from build123d import *

# Parameters (mm, degrees)
SKETCH1_R           = 1.778
BOSS_EXTRUDE1_DEPTH = 152.4
SKETCH2_R           = 2.794
SKETCH2_W           = 25.4
SKETCH2_H           = 6.35
CUT_EXTRUDE1_DEPTH  = 914.4
LPATTERN1_COUNT     = 4
LPATTERN1_PITCH     = 50.8
LPATTERN2_COUNT     = 4
LPATTERN2_PITCH     = 50.8


with BuildPart() as part:
    # Sketch1 → Boss-Extrude1 (new body, symmetric)
    with BuildSketch(Plane(origin=(0, 0, 0), x_dir=(0, 0, -1), z_dir=(1, 0, 0))):
        with BuildLine():
            Line((0, -2.794), (25.4, -2.794))
            Line((25.4, -2.794), (25.4, -1.778))
            Line((25.4, -1.778), (2.155261469, -1.778))
            ThreePointArc((2.155261469, -1.778), (-1.191365603, 2.52726809), (0, -2.794))
        make_face()
        Circle(SKETCH1_R, mode=Mode.SUBTRACT)
    extrude(amount=BOSS_EXTRUDE1_DEPTH, both=True)

    # Sketch2 → Cut-Extrude1 (cut, symmetric)
    with BuildSketch(Plane(origin=(0, -1.778, 0), x_dir=(1, 0, 0), z_dir=(0, 1, 0))):
        with Locations((-25.4, 14.224)):
            Circle(SKETCH2_R)
        with Locations((-12.7, 0.381)):
            Rectangle(SKETCH2_W, SKETCH2_H)
    cut_extrude1 = extrude(amount=CUT_EXTRUDE1_DEPTH, both=True, mode=Mode.SUBTRACT)

    # LPattern1: Cut-Extrude1 ×4
    with Locations(*[(-i * LPATTERN1_PITCH, 0, 0) for i in range(1, LPATTERN1_COUNT)]):
        add(cut_extrude1, mode=Mode.SUBTRACT)

    # LPattern2: Cut-Extrude1 ×4
    with Locations(*[(i * LPATTERN2_PITCH, 0, 0) for i in range(1, LPATTERN2_COUNT)]):
        add(cut_extrude1, mode=Mode.SUBTRACT)


solid = part.part
Model file for the job. Use its own axes, mm. A direction names the side the tool comes from. Round coordinates to 2 decimals unless told otherwise and drop trailing zeros. Loops run counter-clockwise (first coordinate to the right, second up) from the corner with the lowest first, then second, coordinate; pieces in that order, holes last. Notation, with made-up numbers: M -31,-38 L 22,-38 A18 ccw 22,-31 Z; hole C 63,31.5 d8. An arc over 180 degrees is marked long. One line per question, with ' | ' between items.
1) Mould opens along Z. For faces 1 (the flat face through (2, -2.794, -13)), 2 (the cylindrical face through (126.394, -2.279, -11.496)) say: +Z half, -Z half, draft (parallel to the pull), parting line (faces both ways), or undercut.
Solved:
face 1: draft | face 2: undercut
2) Band-saw the part on A-A (z = -22.25). Give the cut face in (x, y).
Solved:
outline: M -152.4,-2.79 L 152.4,-2.79 L 152.4,-1.78 L -152.4,-1.78 Z
3) Drill centre lines: line 1 along X through (y, z) = (-1.9, 1.5); line 2 along Y through (x, z) = (118.5, 0). Where is each one in solid material? Low to high.
Solved:
line 1: x = -152.4 to -127, -101.6 to -76.2, -50.8 to -25.4, 0 to 25.4, 50.8 to 76.2, 101.6 to 127 | line 2: y = -2.79 to -1.78, 1.78 to 2.79
4) Flat gauge pins, fed straight in: pin 1 (3 mm diameter, centred on y = 0, z = 0, fed in from +X); pin 2 (3 mm diameter, centred on y = 1, z = 0, fed in from +X); pin 3 (0.5 mm diameter, centred on x = -14, y = -2.5, fed in from +Z); pin 4 (9 mm diameter, centred on x = -76.2, z = -14.224, fed in from -Y). Where does each tip first touch, or does it go through?
Solved:
pin 1: passes through | pin 2: stops at x = 127 | pin 3: stops at z = -3.56 | pin 4: stops at y = -2.79
5) Band-saw the part on B-B (x = 43.5). Give the cut face in (y, z).
Solved:
outline: M -2.79,-25.4 L -1.78,-25.4 L -1.78,-3.56 L -2.79,-3.56 Z
6) 3-axis set-ups, long thin cutter, end or side, ignore diameter. For faces 3 (the flat face through (-25.4, -1, -2)), 4 (the flat face through (127, -1, -2)), 5 (the cylindrical face through (-78.99, -2.28, -14.35)): which of +Z, -Z, +X, -X, +Y, -Y reach the whole face in a straight line?
Solved:
face 3: +Z, +Y, -Y | face 4: +Z, +X, +Y, -Y | face 5: +Y, -Y
